Here's how the part is built. I have some questions about the finished solid (model axes, mm). Face numbers are marked on the shaded views. Round coordinates to 2 decimals unless told otherwise and drop trailing zeros. Loops run counter-clockwise (first coordinate to the right, second up) from the corner with the lowest first, then second, coordinate; pieces in that order, holes last. Notation, with made-up numbers: (40.25, 61.25) -> (73.25, 61.25) arc R16 cw to (73.25, 90.25) -> close; hole circle Ø10 at (50, 67.25). An arc over 180 degrees is marked (long way). Use CSV: the item, a comma, the result in double quotes. Start each with the question number.
from build123d import *

# Parameters (mm, degrees)
F1_DEPTH = 16
F3_D     = 4


# Not quite as in the source:
# - a feature of the source that left no trace in its solid (it failed there, or was rolled back) is left out
# - the program builds the solid bodies; features that only make, move or delete a surface that nothing else refers to are left out


with BuildPart() as f1:
    # F0 (on Front) → F1 (new body)
    with BuildSketch(Plane.XZ):
        with BuildLine():
            ThreePointArc((-10.8166538264, 0), (0, 9), (10.8166538264, 0))
            Line((10.8166538264, 0), (20, 0))
            Line((20, 0), (20, 17))
            Line((20, 17), (-20, 17))
            Line((-20, 17), (-20, 0))
            Line((-20, 0), (-10.8166538264, 0))
        make_face()
    extrude(amount=F1_DEPTH)

    # F3 (through all)
    with Locations(Plane.XY.offset(17)):
        with Locations((13, -9), (-13, -9)):
            Hole(F3_D / 2)


solid = f1.part
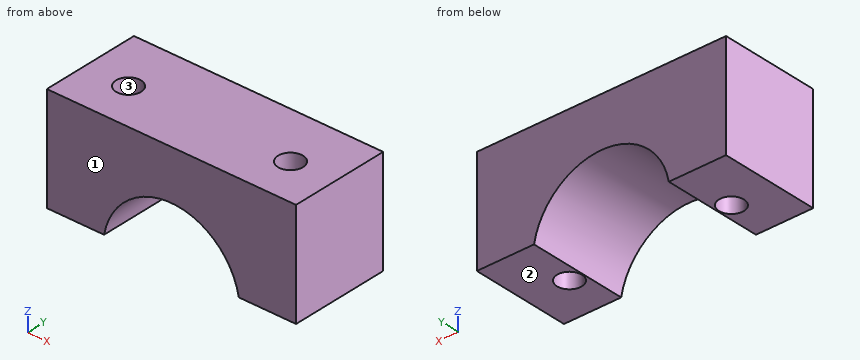
Q1. I need wall thicknesses on line 1 along Y through (x, z) = (13, 11); line 2 along X through (y, z) = (-10.5, 5.5); line 3 along X through (y, z) = (-14.5, 5). Which ranges of each line are inside material? Lowest first, please.
Q2. I want a section at C-C, the plane z = 3. List the corners of the cut face in (x, y) for me.
Q3. Will these pins go through, and if not, where does the flat tip stop? pin 1 Ø6 at (x, y) = (4, -11.5) entering from -Z; pin 2 Ø3 at (x, y) = (-13, -9) entering from +Z.
Q4. I want a section at A-A, the plane y = -9. List the corners of the cut face in (x, z) for me, then the cut area to 3 significant figures.
Q5. I want a section at B-B, the plane x = -13. List the corners of the cut face in (y, z) for me.
Q6. I want a section at D-D, the plane z = 10.25. List the corners of the cut face in (x, y) for me.
Q7. If we mould it in two halves opening along Y, with no side actions, what happens to the marked faces 1, 2 and 3? For each: pulls with the +Y half, pulls with the -Y half, needs draft (parallel to the pull), parting line crosses it, or undercut.
Values found:
1,line 1,"-16 to -11, -7 to 0"
1,line 2,"-20 to -14.32, -11.68 to -8.05, 8.05 to 11.68, 14.32 to 20"
1,line 3,"-20 to -8.49, 8.49 to 20"
2,outline,"(-20, -16) -> (-9.8, -16) -> (-9.8, 0) -> (-20, 0) -> close; (9.8, -16) -> (20, -16) -> (20, 0) -> (9.8, 0) -> close; hole circle Ø4 at (-13, -9); hole circle Ø4 at (13, -9)"
3,pin 1,"z = 6.49"
3,pin 2,"through"
4,outline,"(-20, 0) -> (-15, 0) -> (-15, 17) -> (-20, 17) -> close; (-11, 0) -> (-10.82, 0) arc R11 cw to (10.82, 0) -> (11, 0) -> (11, 17) -> (-11, 17) -> close; (15, 0) -> (20, 0) -> (20, 17) -> (15, 17) -> close"
4,area,"398 mm2"
5,outline,"(-16, 0) -> (-11, 0) -> (-11, 17) -> (-16, 17) -> close; (-7, 0) -> (0, 0) -> (0, 17) -> (-7, 17) -> close"
6,outline,"(-20, -16) -> (20, -16) -> (20, 0) -> (-20, 0) -> close; hole circle Ø4 at (-13, -9); hole circle Ø4 at (13, -9)"
7,face 1,"pulls with the -Y half"
7,face 2,"needs draft"
7,face 3,"undercut"
